Check sheet for the modelled part. Datum: model origin and axes. Units: mm. Face numbers are marked on the shaded views. Give positions to 0.01 mm unless a question says otherwise; leave off trailing zeros. Loops run counter-clockwise (first coordinate to the right, second up) from the corner with the lowest first, then second, coordinate; pieces in that order, holes last. Notation, with made-up numbers: M 16,-36 L 60,-36 A26 cw 60,1 Z; hole C 84,56 d10. An arc over 180 degrees is marked long. Put each result on its own line as item: value. Start each with the question number.
```python
from build123d import *

# Parameters (mm, degrees)
F1_DEPTH = 35


with BuildPart() as f1:
    # F0 (on Front) → F1 (new body)
    with BuildSketch(Plane.XZ):
        with BuildLine():
            Line((6.706351, 0), (3.206351, 0))
            ThreePointArc((3.206351, 0), (4.315396, -2.556039), (6.939684, -3.492214))
            Line((6.939684, -3.492214), (29.339684, -1.995551))
            ThreePointArc((29.339684, -1.995551), (30.666944, -1.36626), (31.206351, 0))
            Line((31.206351, 0), (29.206351, 0))
            Line((29.206351, 0), (6.706351, 0))
        make_face()
        with BuildLine():
            ThreePointArc((6.939684, 3.492214), (4.315396, 2.556039), (3.206351, 0))
            Line((3.206351, 0), (6.706351, 0))
            Line((6.706351, 0), (29.206351, 0))
            Line((29.206351, 0), (31.206351, 0))
            ThreePointArc((31.206351, 0), (30.666944, 1.36626), (29.339684, 1.995551))
            Line((29.339684, 1.995551), (6.939684, 3.492214))
        make_face()
        with BuildLine():
            Line((-0.793649, 0), (-5.793649, 0))
            ThreePointArc((-5.793649, 0), (-4.209299, -3.651484), (-0.460316, -4.988877))
            Line((-0.460316, -4.988877), (29.406351, -2.993326))
            ThreePointArc((29.406351, -2.993326), (31.397241, -2.04939), (32.206351, 0))
            Line((32.206351, 0), (31.206351, 0))
            ThreePointArc((31.206351, 0), (30.666944, -1.36626), (29.339684, -1.995551))
            Line((29.339684, -1.995551), (6.939684, -3.492214))
            ThreePointArc((6.939684, -3.492214), (4.315396, -2.556039), (3.206351, 0))
            Line((3.206351, 0), (-0.793649, 0))
        make_face()
        with BuildLine():
            ThreePointArc((-0.460316, 4.988877), (-4.209299, 3.651484), (-5.793649, 0))
            Line((-5.793649, 0), (-0.793649, 0))
            Line((-0.793649, 0), (3.206351, 0))
            ThreePointArc((3.206351, 0), (4.315396, 2.556039), (6.939684, 3.492214))
            Line((6.939684, 3.492214), (29.339684, 1.995551))
            ThreePointArc((29.339684, 1.995551), (30.666944, 1.36626), (31.206351, 0))
            Line((31.206351, 0), (32.206351, 0))
            ThreePointArc((32.206351, 0), (31.397241, 2.04939), (29.406351, 2.993326))
            Line((29.406351, 2.993326), (-0.460316, 4.988877))
        make_face()
    extrude(amount=-F1_DEPTH)


solid = f1.part
```
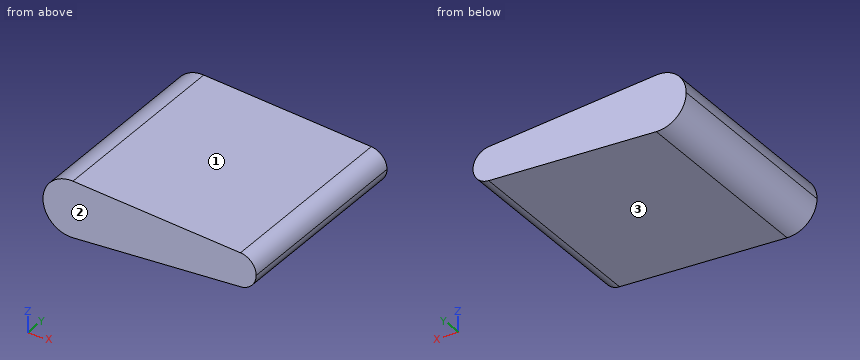
Q1. Mould release check, pull along Z, two halves, no side actions. Record for the marked faces 1, 2 and 3: pulls with the +Z half, pulls with the -Z half, needs draft (parallel to the pull), parting line crosses it, or undercut.
Q2. Depth check by flat-ended pin: P1, Ø4, axis at x = 6.5, y = 20.5, coming from the -Z side; P2, Ø1, axis at x = 1.5, y = 25, coming from the -Z side; P3, Ø4, axis at x = 22.5, y = 22, coming from the +Z side. Enter the tip coordinate at first touch or a pass-through.
Q3. Section check B-B, the plane x = 6. Record the cut outline in (y, z), then the cut area to 3 significant figures.
Q4. Thickness scan on line 1 along Z through (x, y) = (-1, 21); line 2 along X through (y, z) = (18, -2.5); line 3 along Z through (x, y) = (1.5, 7). Record the ranges inside material, lowest first. Write a range as [from, to].
Q5. Section check C-C, the plane z = 3.75. Record the cut outline in (x, y).
Q6. Section check A-A, the plane y = 10.5. Record the cut outline in (x, z).
Found:
1. face 1: pulls with the +Z half
1. face 2: needs draft
1. face 3: pulls with the -Z half
2. P1: stops at z = -4.66
2. P2: stops at z = -4.89
2. P3: stops at z = 3.59
3. outline: M 0,-4.56 L 35,-4.56 L 35,4.56 L 0,4.56 Z
3. area: 319 mm^2
4. line 1: z = [-5, 5]
4. line 2: x = [-5.12, 30.86]
4. line 3: z = [-4.86, 4.86]
5. outline: M -4.1,0 L 18.08,0 L 18.08,35 L -4.1,35 Z
6. outline: M -0.46,-4.99 L 29.41,-2.99 A3 ccw 32.21,0 A3 ccw 29.41,2.99 L -0.46,4.99 A5 ccw long Z
